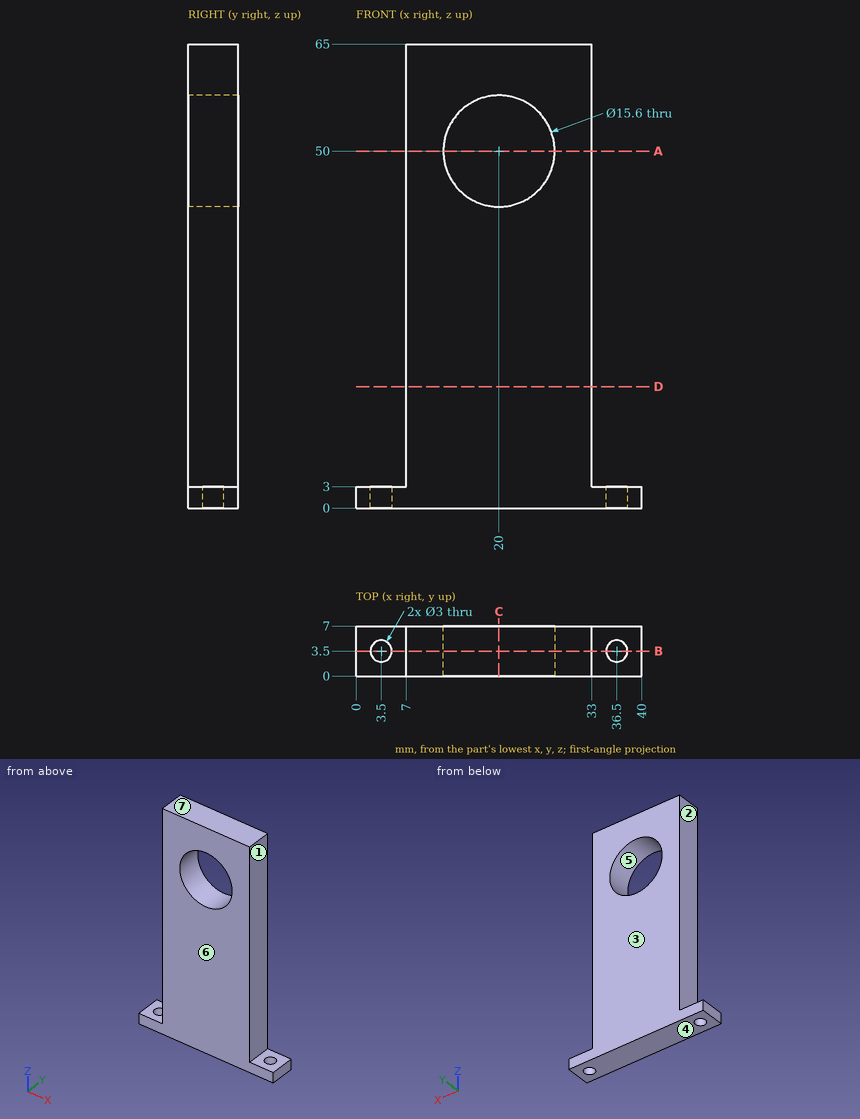
Study the drawing (mm; zero at the part's minimum x, y, z) and answer. A direction names the side the tool comes from. Coordinates: 2 decimals unless noted, no trailing zeros. Write each loop counter-clockwise with the first axis right and the second up, starting at its lowest first coordinate (ties: lowest second). Pieces come first, ordered by that corner, then holes. Notation, with made-up numbers: (-8.75, 4) - (31.25, 4) arc R36 ccw to (31.25, 39) - close; hole circle Ø8 at (31, 50). An arc over 180 degrees is marked (long way). Return JSON: item names as keys, results as strings. Group by question number.
1. A cutting plane is placed at B-B, the plane y = 3.5. Determine the outline of the cut face in (x, z), plus the area to 3 significant figures.
2. A cutting plane is placed at A-A, the plane z = 50. Determine the outline of the cut face in (x, y).
3. Given pin 1 (4 mm diameter, centred on x = 13.5, z = 47, fed in from +Y); pin 2 (8 mm diameter, centred on x = 20.5, z = 49, fed in from +Y); pin 3 (3.5 mm diameter, centred on x = 4.5, y = 3, fed in from +Z), each flat-ended and moving along its own axis, determine where each tip first touches the part or whether it passes through.
4. A cutting plane is placed at D-D, the plane z = 17. Determine the outline of the cut face in (x, y).
5. Which of the six approach directions +Z, -Z, +X, -X, +Y, -Y give full straight-line access (tool end or side, diameter ignored) to the marked faces 1, 2 and 3?
6. Determine the mould class of the marked faces 4, 5, 6 and 7 for opening direction Z: released by +Z, released by -Z, zero draft, split by the parting line, or undercut.
7. A cutting plane is placed at C-C, the plane x = 20. Determine the outline of the cut face in (y, z), plus the area to 3 significant figures.
8. Straight lines are drawn through the part: L1, parallel to Y at x = 36.5, z = 1; L2, parallel to X at y = 2, z = 38; L3, parallel to Z at x = 33.5, y = 5.5. For each, find the intervals that lie inside material, in ascending order.
Ans:
{
 "1": {"outline": "(0, 0) - (2, 0) - (2, 3) - (0, 3) - close; (5, 0) - (35, 0) - (35, 3) - (33, 3) - (33, 65) - (7, 65) - (7, 3) - (5, 3) - close; (38, 0) - (40, 0) - (40, 3) - (38, 3) - close; hole circle Ø15.6 at (20, 50)", "area": "1,520 mm²"},
 "2": {"outline": "(7, 0) - (12.2, 0) - (12.2, 7) - (7, 7) - close; (27.8, 0) - (33, 0) - (33, 7) - (27.8, 7) - close"},
 "3": {"pin 1": "y = 7", "pin 2": "through", "pin 3": "z = 3"},
 "4": {"outline": "(7, 0) - (33, 0) - (33, 7) - (7, 7) - close"},
 "5": {"face 1": "+Z, +X, +Y, -Y", "face 2": "+Z, -X, +Y, -Y", "face 3": "+Z, -Z, +X, -X, +Y"},
 "6": {"face 4": "released by -Z", "face 5": "undercut", "face 6": "zero draft", "face 7": "released by +Z"},
 "7": {"outline": "(0, 0) - (7, 0) - (7, 42.2) - (0, 42.2) - close; (0, 57.8) - (7, 57.8) - (7, 65) - (0, 65) - close", "area": "346 mm²"},
 "8": {"L1": "0 to 2, 5 to 7", "L2": "7 to 33", "L3": "0 to 3"}
}
